Autodesk Inventor part; units mm, degrees
ref_plane "YZ Plane" through (0, 0, 0) normal (1, 0, 0) x (0, 1, 0)
ref_plane "XZ Plane" through (0, 0, 0) normal (0, 1, 0) x (-1, 0, 0)
ref_plane "XY Plane" through (0, 0, 0) normal (0, 0, 1) x (1, 0, 0)
sketch "Sketch3" plane through (0, 0, 0) normal (0, 1, 0) x (-1, 0, 0)
  line L0 (0, 0) -> (70, 0)
  line L1 (70, 0) -> (70, -70)
  line L2 (70, -70) -> (70, -94)
  line L3 (70, -94) -> (64, -94)
  line L4 (64, -94) -> (64, -70)
  line L5 (64, -3) -> (0, -3)
  line L6 (0, -3) -> (0, 0)
  line L7 (64, -70) -> (67, -70)
  line L8 (67, -70) -> (67, -3)
  line L9 (67, -3) -> (64, -3)
  circle A0 centre (67, -82) radius 2.125
  circle A1 centre (67, -76) radius 2.125
  circle A2 centre (67, -88) radius 2.125
  dimension "d26" = 70
  dimension "d27" = 70
  dimension "d29" = 6
  dimension "d55" = 4.25
  dimension "d56" = 4.25
  dimension "d57" = 4.25
  dimension "d59" = 6
  dimension "d60" = 6
  dimension "d61" = 6
extrude "Extrusion2" add sketch "Sketch3" along normal blind 27 contours L0 L1 L2 L3 L4 L7 L8 L9 L5 L6 | A0 | A1 | A2
sketch "Sketch4" plane through (0, 27, 0) normal (0, 1, 0) x (1, 0, 0)
  line L0 (-70, 0) -> (0, 0)
  line L1 (0, 0) -> (0, 3)
  line L2 (-70, 0) -> (0, 0)
  line L3 (0, 0) -> (0, 3)
  line L4 (0, 3) -> (-70, 3)
  line L5 (-70, 3) -> (-70, 0)
extrude "Extrusion3" add sketch "Sketch4" along normal blind 20
sketch "Sketch5" plane through (-70, 0, -94) normal (-1, 0, 0) x (0, 0, 1)
  line L0 (-0.1204, 1.5) -> (23.8796, 1.5)
  line L1 (23.8796, 1.5) -> (23.8796, 25.5)
  line L2 (23.8796, 25.5) -> (-0.1204, 25.5)
  line L3 (-0.1204, 25.5) -> (-0.1204, 1.5)
  line L4 (94, 0) -> (0, 0)
  dimension "d36" = 24
  dimension "d37" = 24
  dimension "d38" = 1.5
extrude "Extrusion4" cut sketch "Sketch5" against normal blind 10
sketch "Sketch9" plane through (0, 0, -3) normal (0, 0, -1) x (-1, 0, 0)
  line L0 (7, 7) -> (60, 7)
  line L1 (60, 7) -> (60, 39)
  line L2 (60, 39) -> (7, 39)
  line L3 (7, 39) -> (7, 7)
  line L4 (0, 0) -> (0, 47)
  line L5 (67, 0) -> (0, 0)
  dimension "d45" = 53
  dimension "d46" = 32
  dimension "d47" = 7
  dimension "d48" = 7
extrude "Extrusion5" cut sketch "Sketch9" against normal blind 10
sketch "Sketch10" plane through (-70, 0, 0) normal (0, 0, 1) x (1, 0, 0)
  line L0 (10, 39) -> (10, 7)
  line L1 (63, 7) -> (63, 39)
  line L2 (63, 26.6385) -> (63, 18.6385)
  line L3 (10, 18.6385) -> (10, 26.6385)
  line L4 (63, 39) -> (10, 39)
  line L5 (10, 7) -> (63, 7)
  line L6 (31.6097, 39) -> (39.6097, 39)
  line L7 (39.6097, 39) -> (39.6097, 7)
  line L8 (39.6097, 7) -> (31.6097, 7)
  line L9 (31.6097, 7) -> (31.6097, 18.6385)
  line L10 (31.6097, 26.6385) -> (31.6097, 39)
  line L11 (10, 26.6385) -> (31.6097, 26.6385)
  line L12 (39.6097, 26.6385) -> (63, 26.6385)
  line L13 (63, 18.6385) -> (39.6097, 18.6385)
  line L14 (31.6097, 18.6385) -> (10, 18.6385)
  point P0 (70, 0)
  dimension "d51" = 8
  dimension "d52" = 8
extrude "Extrusion6" add sketch "Sketch10" against normal blind 3 contours L11 L10 L4 L7 L5 L9 L14 L0 | L12 L1 L13 L7
sketch "Sketch11" plane through (0, 0, 0) normal (0, -1, 0) x (1, 0, 0)
  point P0 (0, 0)
sketch "Sketch12" plane through (0, 0, 0) normal (0, -1, 0) x (1, 0, 0)
  circle A0 centre (-67, -82) radius 2.125
  circle A1 centre (-67, -76) radius 2.125
  circle A2 centre (-67, -88) radius 2.125
  line L0 (-64, -70) -> (-67, -70)
  point P0 (0, 0)
  dimension "d62" = 4.25
  dimension "d63" = 4.25
  dimension "d64" = 4.25
  dimension "d65" = 6
  dimension "d66" = 6
  dimension "d67" = 6
hole "Hole2" at (-67, 0, -88) at (-67, 0, -82) at (-67, 0, -76) direction (0, 1, 0) diameter 4.25 end through all
sketch "Sketch13" plane through (-70, 0, -94) normal (-1, 0, 0) x (0, 0, 1)
  point P0 (94, 0)
properties part number "GrapperRight"
Could you check a few things on this model? Use its own coordinates, in mm. A direction names the side the tool comes from. Give positions to 0.01 mm unless a question says otherwise; leave off trailing zeros. Order: outer loops, then holes, each group sorted by start corner. A loop starts at its lowest first (then second) coordinate and runs counter-clockwise, first axis right, second up. Notation, with made-up numbers: (-9, -10) - (24, -10) arc R36 ccw to (24, 29) - close; hole circle Ø8 at (-32.75, 80.25). An arc over 180 degrees is marked (long way). One line per question, with ' | ' between items. Start each with the question number.
Item 1: Thinking about a two-plate mould opening in Y: for faces 1 (the cylindrical face through (-68.4, 0.8, -74.4)), 2 (the flat face through (-68, 27, -48)), 3 (the flat face through (-49, 39, -2)), which applies, pulls with the +Y half, pulls with the -Y half, needs draft (parallel to the pull), parting line crosses it, or undercut?
Item 2: I want a section at D-D on z = -64. Write out the boundary of the cut face in (x, y).
Item 3: For faces 4 (the flat face through (-70, 13, -37)), 5 (the flat face through (-7, 13, -2)), 6 (the flat face through (-67, 25.5, -79)), 7 (the flat face through (-67, 13, -37)), 8 (the flat face through (-64, 1, -82)), which set-ups out of +Z, -Z, +X, -X, +Y, -Y let a thin tool reach every point of the face, with its end or its side?
Item 4: I need wall thicknesses on probe 1 along X at (y, z) = (26.5, -82) (3 decimals); probe 2 along Z at (x, y) = (-62, 23); probe 3 along X at (y, z) = (6, -29). Which ranges of each line are inside material? Lowest first, please. Write a range as [from, to].
Item 5: I want a section at A-A on y = 29. Write out the boundary of the cut face in (x, z).
Item 6: I want a section at C-C on y = 24. Write out the boundary of the cut face in (x, z), then the cut area to 3 significant figures.
Item 7: I want a section at B-B on z = -88. Write out the boundary of the cut face in (x, y) (3 decimals), then the cut area to 3 significant figures.
Item 8: I'm going to push flat-ended pins straight in: pin 1 Ø19 at (y, z) = (20, -82) entering from +X; pin 2 Ø13.5 at (y, z) = (11.5, -23.5) entering from +X; pin 3 Ø5 at (x, z) = (-67, -88) entering from +Y. Where does each tip first touch, or does it pass through?
Verdict:
1) face 1: needs draft | face 2: pulls with the +Y half | face 3: undercut
2) outline: (-70, 0) - (-67, 0) - (-67, 27) - (-70, 27) - close
3) face 4: +Z, -Z, -X, +Y, -Y | face 5: +Z, -Z | face 6: -Z, +X, -X | face 7: +X, +Y, -Y | face 8: -Z, +X, +Y, -Y
4) probe 1: [-70, -69.125], [-64.875, -64] | probe 2: [-3, 0] | probe 3: [-70, -67]
5) outline: (-70, -3) - (-60, -3) - (-60, 0) - (-70, 0) - close; (-38.39, -3) - (-30.39, -3) - (-30.39, 0) - (-38.39, 0) - close; (-7, -3) - (0, -3) - (0, 0) - (-7, 0) - close
6) outline: (-70, -70.12) - (-64, -70.12) - (-64, -70) - (-67, -70) - (-67, -3) - (0, -3) - (0, 0) - (-70, 0) - close | area: 412 mm^2
7) outline: (-70, 0) - (-69.125, 0) - (-69.125, 1.5) - (-70, 1.5) - close; (-70, 25.5) - (-69.125, 25.5) - (-69.125, 27) - (-70, 27) - close; (-64.875, 0) - (-64, 0) - (-64, 1.5) - (-64.875, 1.5) - close; (-64.875, 25.5) - (-64, 25.5) - (-64, 27) - (-64.875, 27) - close | area: 5.25 mm^2
8) pin 1: x = -64 | pin 2: x = -67 | pin 3: y = 27
